Read the model definition and answer for the solid it produces. Units are mm, in the model's axes. Round coordinates to 2 decimals unless told otherwise and drop trailing zeros. Order: outer loops, then holes, each group sorted by start corner. A loop starts at its lowest first (then second) coordinate and runs counter-clockwise, first axis right, second up. Notation, with made-up numbers: (71.5, -34.75) - (75.5, -34.75) arc R28 ccw to (75.5, 3.25) - close; hole circle Ø5 at (83.25, -37). An arc over 180 degrees is marked (long way). One line per question, with ' | ' between items. Start each with the question number.
1) The part is cut by section D-D, the plane y = -87. Give the vertices of the cut face in (x, z) (3 decimals), plus the area to 3 significant figures.
2) A flat-ended cylindrical pin translates along its axis: pin 1 (12 mm diameter, centred on x = 22.5, y = -69, fed in from +Z) (3 decimals). Find the tip coordinate at first contact, or state that the pin passes through.
3) The part is cut by section B-B, the plane x = 20. Give the vertices of the cut face in (y, z) (3 decimals).
4) The part is cut by section A-A, the plane x = 42. Give the vertices of the cut face in (y, z) (3 decimals).
5) The part is cut by section C-C, the plane y = -14.5. Give the vertices of the cut face in (x, z) (3 decimals).
from build123d import *

# Parameters (mm, degrees)
SKETCH_W         = 3.322
SKETCH_H         = 8.904724
EXTRUDE003_DEPTH = 0.035
EXTRUDE_DEPTH    = 0.035


with BuildPart() as obj1:
    # Sketch (on Face6 of Extrude001) → Extrude003 (new body)
    with BuildSketch(Plane.XY):
        with Locations((25.530795, 3.517178)):
            Rectangle(SKETCH_W, SKETCH_H)
    extrude(amount=EXTRUDE003_DEPTH)


with BuildPart() as copper_layer:
    # Sketch006 → Extrude (new body)
    with BuildSketch(Plane.XY):
        Polygon((23.498381, -102.062126), (28.273891, -102.062126), (28.273891, -50.486412), (51.949276, -52.498531), (51.949276, -44.41013), (29.665995, -46.231361), (38.564362, -34.246563), (43.545963, -23.426317), (43.545963, -10.302752), (35.56469, -2.321481), (28.543734, 0), (23.13361, 0), (15.098775, -3.218604), (9.045863, -10.985613), (7.920988, -19.074015), (10.759965, -29.626432), (22.596775, -46.640076), (0, -44.497452), (0, -52.63942), (23.498381, -50.665943), align=None)
        with BuildLine():
            Line((12.900836, -18.866589), (13.548023, -24.306177))
            Line((13.548023, -24.306177), (14.994295, -28.698555))
            Line((14.994295, -28.698555), (17.886837, -34.001549))
            Line((17.886837, -34.001549), (25.760977, -42.946999))
            Line((25.760977, -42.946999), (30.314053, -38.340359))
            Line((30.314053, -38.340359), (33.956512, -33.519459))
            Line((33.956512, -33.519459), (37.277576, -27.091587))
            Line((37.277576, -27.091587), (39.221496, -19.680452))
            Line((39.221496, -19.680452), (39.317309, -17.981558))
            Line((39.317309, -17.981558), (39.421192, -16.139563))
            ThreePointArc((39.421192, -16.139563), (38.632704, -13.668833), (37.394095, -11.390222))
            Line((35.933163, -8.951125), (37.394095, -11.390222))
            Line((35.933163, -8.951125), (35.047039, -7.469805))
            ThreePointArc((35.047039, -7.469805), (20.72172, -5.915046), (12.85167, -17.985437))
            Line((12.900836, -18.866589), (12.85167, -17.985437))
        make_face(mode=Mode.SUBTRACT)
    extrude(amount=EXTRUDE_DEPTH)

    # Fusion: union obj1
    add(obj1.part)


solid = copper_layer.part
Values:
1) outline: (23.498, 0) - (28.274, 0) - (28.274, 0.035) - (23.498, 0.035) - close | area: 0.167 mm^2
2) pin 1: stops at z = 0.035
3) outline: (-50.96, 0) - (-46.394, 0) - (-46.394, 0.035) - (-50.96, 0.035) - close; (-42.908, 0) - (-36.402, 0) - (-36.402, 0.035) - (-42.908, 0.035) - close; (-6.283, 0) - (-1.255, 0) - (-1.255, 0.035) - (-6.283, 0.035) - close
4) outline: (-51.653, 0) - (-45.223, 0) - (-45.223, 0.035) - (-51.653, 0.035) - close; (-26.784, 0) - (-8.757, 0) - (-8.757, 0.035) - (-26.784, 0.035) - close
5) outline: (8.557, 0) - (13.399, 0) - (13.399, 0.035) - (8.557, 0.035) - close; (38.956, 0) - (43.546, 0) - (43.546, 0.035) - (38.956, 0.035) - close
